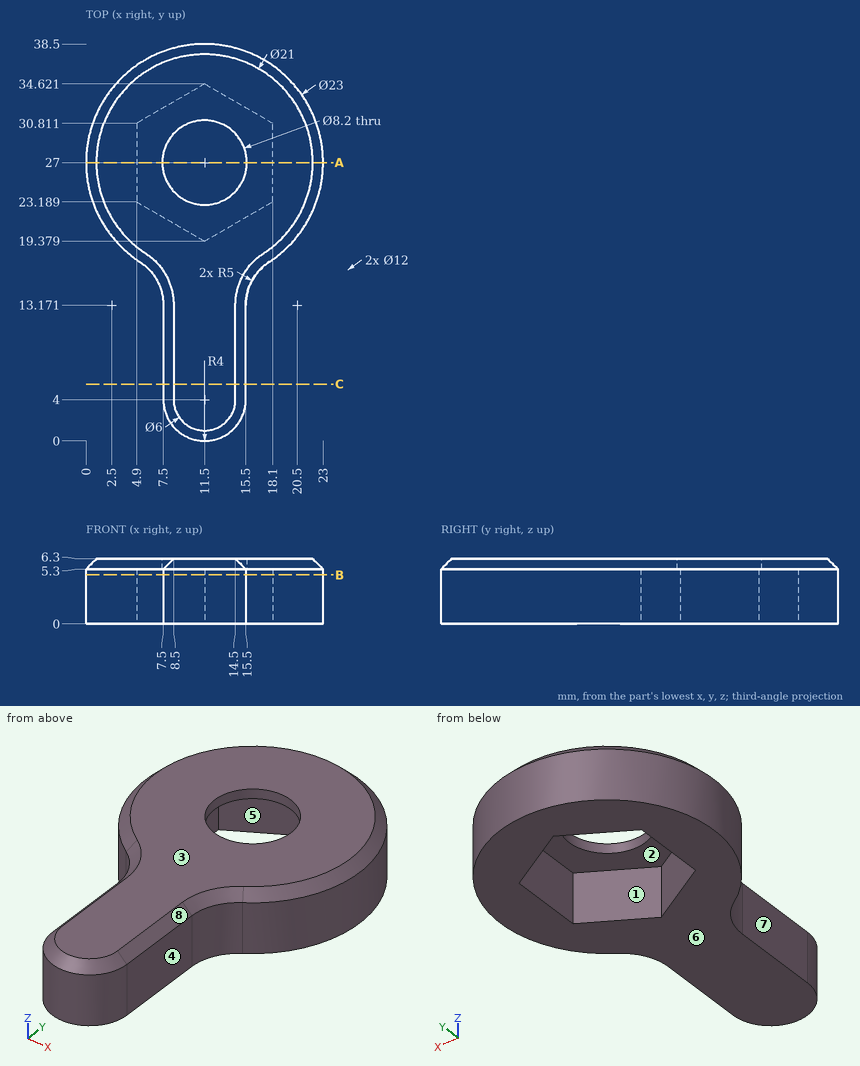
Input: dimensioned drawing with shaded views. Units: mm. Origin: part minimum x, y, z. A direction names the side the tool comes from. Round coordinates to 2 decimals unless told otherwise and drop trailing zeros. Loops run counter-clockwise (first coordinate to the right, second up) from the corner with the lowest first, then second, coordinate; pieces in that order, holes last. Notation, with made-up numbers: (12.5, 36.5) -> (39.5, 36.5) arc R25 cw to (39.5, 68.5) -> close; hole circle Ø7 at (65, 80.5). An arc over 180 degrees is marked (long way). Answer as a JSON object with one key per item and string values. Group by question number.
Q1. Ray query, line 1 (Y direction, x = 11.5, z = 5.75); line 2 (Z direction, x = 6.75, y = 28); line 3 (Y direction, x = 9.25, z = 3.25) (1 decimal). Return the intervals inside material, ascending. Write a range as from..to.
Q2. Mould query, pull axis X, two halves, no side actions, for the marked faces 1, 2, 3 and 4. Classes: pulls with the +X half, pulls with the -X half, needs draft (parallel to the pull), parting line crosses it, or undercut.
Q3. Contact query for flat-ended pins moving along their axis: P1, Ø6.5, axis at x = 13, y = 26, coming from the -Z side; P2, Ø2, axis at y = 8.5, z = 4.5, coming from the +X side; P3, Ø1.6, axis at y = 7.5, z = 3, coming from the -X side. Output: stop coordinate, or through.
Q4. Section query C-C (y = 5.5). Output: boundary loops of the cut face in (x, z), plus the area to 3 significant figures.
Q5. Section query B-B (z = 4.75). Output: boundary loops of the cut face in (x, y).
Q6. Access query for the marked faces 5, 6, 7 and 8. Directions: +Z, -Z, +X, -X, +Y, -Y. A direction counts if a zero-diameter tool reaches every point of the face in a straight line with its end or side. Return the directions, or none.
Q7. Section query A-A (y = 27). Output: boundary loops of the cut face in (x, z).
Completed:
{
 "1": {"line 1": "0.45..22.9, 31.1..38.05", "line 2": "5.3..6.3", "line 3": "0.7..20.7, 33.3..38.3"},
 "2": {"face 1": "undercut", "face 2": "undercut", "face 3": "needs draft", "face 4": "pulls with the +X half"},
 "3": {"P1": "z = 5.3", "P2": "x = 15.5", "P3": "x = 7.5"},
 "4": {"outline": "(7.5, 0) -> (15.5, 0) -> (15.5, 5.3) -> (14.5, 6.3) -> (8.5, 6.3) -> (7.5, 5.3) -> close", "area": "49.4 mm²"},
 "5": {"outline": "(5.23, 17.36) arc R5 cw to (7.5, 13.17) -> (7.5, 4) arc R4 ccw to (15.5, 4) -> (15.5, 13.17) arc R5 cw to (17.77, 17.36) arc R11.5 ccw (long way) to start; hole (4.9, 23.19) -> (11.5, 19.38) -> (18.1, 23.19) -> (18.1, 30.81) -> (11.5, 34.62) -> (4.9, 30.81) -> close"},
 "6": {"face 5": "-Z", "face 6": "-Z, +X, -X, +Y, -Y", "face 7": "+Z, -Z, -X, -Y", "face 8": "+Z, +X, -Y"},
 "7": {"outline": "(0, 0) -> (4.9, 0) -> (4.9, 5.3) -> (7.4, 5.3) -> (7.4, 6.3) -> (1, 6.3) -> (0, 5.3) -> close; (15.6, 5.3) -> (18.1, 5.3) -> (18.1, 0) -> (23, 0) -> (23, 5.3) -> (22, 6.3) -> (15.6, 6.3) -> close"}
}
